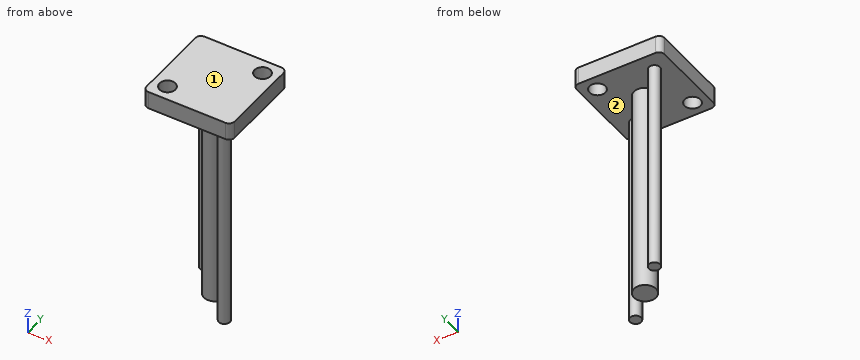
from build123d import *

# Parameters (mm, degrees)
SKETCH1_R           = 5
BOSS_EXTRUDE1_DEPTH = 97
SKETCH2_R           = 3.6
BOSS_EXTRUDE2_DEPTH = 8
BOSS_EXTRUDE3_REACH = 107
SKETCH4_R           = 2.55


with BuildPart() as part:
    # Sketch1 → Boss-Extrude1 (new body)
    with BuildSketch(Plane.XY):
        Circle(SKETCH1_R)
    extrude(amount=BOSS_EXTRUDE1_DEPTH)

    # Sketch2 → Boss-Extrude2 (add)
    with BuildSketch(Plane.XY.offset(97)):
        with BuildLine():
            Line((-17.4, -19.9), (17.4, -19.9))
            ThreePointArc((17.4, -19.9), (19.167766953, -19.167766953), (19.9, -17.4))
            Line((19.9, -17.4), (19.9, 17.4))
            ThreePointArc((19.9, 17.4), (19.167766953, 19.167766953), (17.4, 19.9))
            Line((17.4, 19.9), (-17.4, 19.9))
            ThreePointArc((-17.4, 19.9), (-19.167766953, 19.167766953), (-19.9, 17.4))
            Line((-19.9, 17.4), (-19.9, -17.4))
            ThreePointArc((-19.9, -17.4), (-19.167766953, -19.167766953), (-17.4, -19.9))
        make_face()
        with Locations((13.15, 13.15)):
            Circle(SKETCH2_R, mode=Mode.SUBTRACT)
        with Locations((-13.15, -13.15)):
            Circle(SKETCH2_R, mode=Mode.SUBTRACT)
    extrude(amount=BOSS_EXTRUDE2_DEPTH)

    # Sketch4 → Boss-Extrude3 (add, up to next)
    with BuildSketch(Plane(origin=(0, 0, 0), x_dir=(-1, 0, 0), z_dir=(0, 0, -1)), mode=Mode.PRIVATE) as boss_extrude3_sk1:
        with Locations((-11.7, -11.7)):
            Circle(SKETCH4_R)
    boss_extrude3_tool1 = extrude(boss_extrude3_sk1.sketch, amount=-BOSS_EXTRUDE3_REACH, mode=Mode.PRIVATE) - part.part
    add(boss_extrude3_tool1.solids().sort_by_distance((11.7, -11.7, 0))[0])
    # Sketch4 → Boss-Extrude3 (add, up to next)
    with BuildSketch(Plane(origin=(0, 0, 0), x_dir=(-1, 0, 0), z_dir=(0, 0, -1)), mode=Mode.PRIVATE) as boss_extrude3_sk2:
        with Locations((11.7, 11.7)):
            Circle(SKETCH4_R)
    boss_extrude3_tool2 = extrude(boss_extrude3_sk2.sketch, amount=-BOSS_EXTRUDE3_REACH, mode=Mode.PRIVATE) - part.part
    add(boss_extrude3_tool2.solids().sort_by_distance((-11.7, 11.7, 0))[0])


solid = part.part
Design review of the part built by this model. Coordinates are the model's own, in mm. Face numbers are marked on the shaded views. A direction names the side the tool comes from. Coordinates: 2 decimals unless noted, no trailing zeros. Order: outer loops, then holes, each group sorted by start corner. A loop starts at its lowest first (then second) coordinate and runs counter-clockwise, first axis right, second up. Notation, with made-up numbers: (60, 28) - (71, 28) arc R19 cw to (71, 48) - close; hole circle Ø8 at (-12.5, 42.5). An arc over 180 degrees is marked (long way). Put each result on its own line as item: value.
1) Insertion check: P1, Ø1.5, axis at x = -10, z = 59.5, coming from the -Y side; P2, Ø5, axis at y = 8, z = 35.5, coming from the -X side; P3, Ø3, axis at x = -11, y = -0.5, coming from the -Z side. Each pin has a flat end and moves straight along its axis. Give the tip position at first contact, or say it passes through.
Response values:
P1: stops at y = 9.33
P2: stops at x = -13.95
P3: stops at z = 97
2) Tool access review of the marked faces 1 and 2: name each direction out of +Z, -Z, +X, -X, +Y, -Y from which nothing blocks a thin tool from reaching the whole face with its end or side.
Response values:
face 1: +Z, +X, -X, +Y, -Y
face 2: -Z
3) Take a section at A-A, the plane x = 11.7. Give the boundary of the cut face in (y, z), and give its area (3 significant figures).
Response values:
outline: (-19.9, 97) - (-14.25, 97) - (-14.25, 0) - (-9.15, 0) - (-9.15, 97) - (9.85, 97) - (9.85, 105) - (-19.9, 105) - close; (16.45, 97) - (19.9, 97) - (19.9, 105) - (16.45, 105) - close
area: 760 mm²
4) Take a section at B-B, the plane y = -11.7. Give the boundary of the cut face in (x, z).
Response values:
outline: (-19.9, 97) - (-16.45, 97) - (-16.45, 105) - (-19.9, 105) - close; (-9.85, 97) - (9.15, 97) - (9.15, 0) - (14.25, 0) - (14.25, 97) - (19.9, 97) - (19.9, 105) - (-9.85, 105) - close
5) Take a section at C-C, the plane z = 25. Give the boundary of the cut face in (x, y).
Response values:
outline: circle Ø5.1 at (-11.7, 11.7); circle Ø10 at (0, 0); circle Ø5.1 at (11.7, -11.7)
6) Wall thickness on L1, parallel to Y at x = 13.15, z = 99; L2, parallel to Y at x = -13.15, z = 100: over which ranges is each line inside the solid? List them lowest first. Write a range as from..to.
Response values:
L1: y = -19.9..9.55, 16.75..19.9
L2: y = -19.9..-16.75, -9.55..19.9
7) Take a section at D-D, the plane x = 0. Give the boundary of the cut face in (y, z).
Response values:
outline: (-19.9, 97) - (-5, 97) - (-5, 0) - (5, 0) - (5, 97) - (19.9, 97) - (19.9, 105) - (-19.9, 105) - close
